Job drawing, mm, ordinate dimensions from the low corner. One solid piece. Round coordinates to 2 decimals unless told otherwise and drop trailing zeros. Write each loop counter-clockwise with the first axis right and the second up, starting at its lowest first coordinate (ties: lowest second). Pieces come first, ordered by that corner, then holes. Notation, with made-up numbers: M 86,61.25 L 134,61.25 A5 ccw 134,69.25 Z; hole C 69,-28 d10. An arc over 180 degrees is marked long. Answer as a JSON object with one key per item and string values. Group by question number.
1. Band-saw the part on A-A, the plane x = 40. Write the cut outline in (y, z), plus the area to 3 significant figures.
2. Two-plate mould, pull along Y, no slides. Class the marked faces 1 and 2: +Y half, -Y half, draft (parallel to the pull), parting line (faces both ways), or undercut.
3. Band-saw the part on C-C, the plane z = 3.2. Count the separate pieces of the cut face and the enclosed holes in it, plus the area to 3 significant figures.
4. Drop a flat-ended pin along its axis: pin 1 (8 mm diameter, centred on x = 28.5, y = 19.5, fed in from -Z). Give the stop position or say it passes through.
5. Band-saw the part on D-D, the plane y = 9. Write the cut outline in (x, z).
6. Drill centre lines: line 1 (Y direction, x = 40, z = 2.7); line 2 (X direction, y = 9.5, z = 2.8) (1 decimal); line 3 (X direction, y = 24, z = 4.1) (1 decimal). Where is each one in solid material? Low to high. Write a range as from..to.
7. Band-saw the part on B-B, the plane y = 20. Write the cut outline in (x, z), plus the area to 3 significant figures.
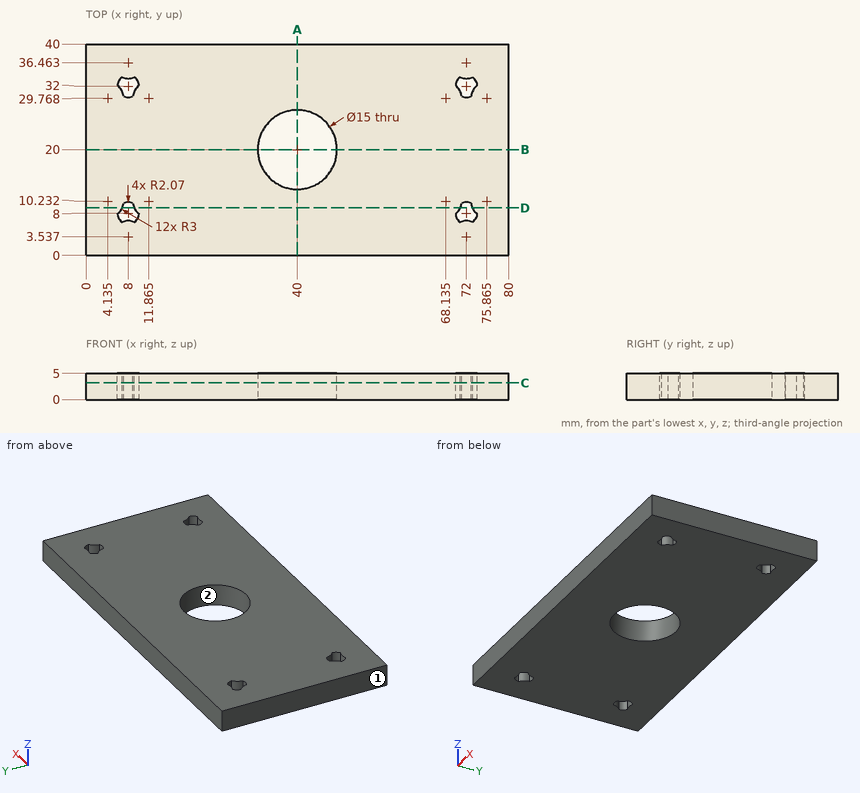
Worked answers:
{
 "1": {"outline": "M 0,0 L 12.5,0 L 12.5,5 L 0,5 Z; M 27.5,0 L 40,0 L 40,5 L 27.5,5 Z", "area": "125 mm^2"},
 "2": {"face 1": "draft", "face 2": "undercut"},
 "3": {"separate pieces": "1", "enclosed holes": "5", "area": "2,980 mm^2"},
 "4": {"pin 1": "stops at z = 0"},
 "5": {"outline": "M 0,0 L 6.87,0 L 6.87,5 L 0,5 Z; M 9.13,0 L 70.87,0 L 70.87,5 L 9.13,5 Z; M 73.13,0 L 80,0 L 80,5 L 73.13,5 Z"},
 "6": {"line 1": "y = 0..12.5, 27.5..40", "line 2": "x = 0..7, 9..71, 73..80", "line 3": "x = 0..33.7, 46.3..80"},
 "7": {"outline": "M 0,0 L 32.5,0 L 32.5,5 L 0,5 Z; M 47.5,0 L 80,0 L 80,5 L 47.5,5 Z", "area": "325 mm^2"}
}
